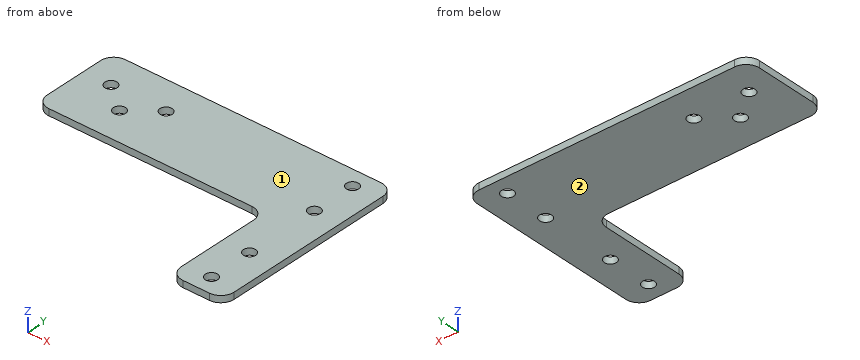
```python
from build123d import *

# Parameters (mm, degrees)
ODGI_CIE_BAZOWE1_DEPTH = 3
OTW_R_POD_RUB_M51_D    = 5.5
ZAOKR_GLENIE1_R        = 6


# Sheet-metal steps are written as plain solids
with BuildPart() as part:
    # Szkic1 → Odgięcie bazowe1 (new body)
    with BuildSketch(Plane.XY):
        Polygon((0, 0), (-104, 0), (-104, 40), (24, 40), (24, -50), (0, -50), align=None)
    extrude(amount=-ODGI_CIE_BAZOWE1_DEPTH)

    # Otwór pod śrubę M51 (through all)
    with Locations(Plane.XY):
        with Locations((12, -42), (12, -22), (12, 12), (12, 32), (-91.5, 25), (-66.5, 25), (-79, 15)):
            Hole(OTW_R_POD_RUB_M51_D / 2)

    # Zaokrąglenie1
    zaokr_glenie1_edges = [part.edges().sort_by_distance(p)[0] for p in [
        (0, 0, -1.5),
        (-104, 0, -1.5),
        (-104, 40, -1.5),
        (24, 40, -1.5),
        (24, -50, -1.5),
        (0, -50, -1.5),
    ]]
    fillet(zaokr_glenie1_edges, radius=ZAOKR_GLENIE1_R)


solid = part.part
```
The listing builds one solid part. Answer for the finished solid, in the listing's coordinates (mm). Face numbers are marked on the shaded views. Give positions to 0.01 mm unless a question says otherwise; leave off trailing zeros. Write each loop counter-clockwise with the first axis right and the second up, starting at its lowest first coordinate (ties: lowest second). Pieces come first, ordered by that corner, then holes. Notation, with made-up numbers: (54, 23) -> (72, 23) arc R29 cw to (72, 44) -> close; hole circle Ø11 at (-39.75, -5). An arc over 180 degrees is marked (long way). Write item = value, one per line. Start each with the question number.
1) The part is cut by section A-A, the plane y = 32. Determine the outline of the cut face in (x, z).
2) Each of these flat-tipped pins is pushed along its axis until it touches: pin 1 (0.9 mm diameter, centred on y = -25, z = -2, fed in from -X); pin 2 (0.9 mm diameter, centred on x = -45.5, z = -2, fed in from -Y). Where does it stop, or does it pass through?
3) The part is cut by section B-B, the plane x = -66.5. Determine the outline of the cut face in (y, z), and give its area (4 significant figures).
4) The part is cut by section D-D, the plane x = 12. Determine the outline of the cut face in (y, z), and give its area (3 significant figures).
5) The part is cut by section C-C, the plane z = -2.2. Determine the outline of the cut face in (x, y), and give its area (3 significant figures).
6) Determine the mould class of the marked faces 1 and 2 for opening direction Z: +Z half, -Z half, draft (parallel to the pull), parting line (faces both ways), or undercut.
7) Straight lines are drawn through the part: line 1 along Y through (x, z) = (12, -2.2); line 2 along Y through (x, z) = (-66.5, -1.75); line 3 along Y through (x, z) = (-21, -2.7). For each, find the intervals that lie inside material, in ascending order.
Solutions:
q1.outline = (-104, -3) -> (9.25, -3) -> (9.25, 0) -> (-104, 0) -> close; (14.75, -3) -> (24, -3) -> (24, 0) -> (14.75, 0) -> close
q2.pin_1 = 0
q2.pin_2 = 0
q3.outline = (0, -3) -> (22.25, -3) -> (22.25, 0) -> (0, 0) -> close; (27.75, -3) -> (40, -3) -> (40, 0) -> (27.75, 0) -> close
q3.area = 103.5 mm²
q4.outline = (-50, -3) -> (-44.75, -3) -> (-44.75, 0) -> (-50, 0) -> close; (-39.25, -3) -> (-24.75, -3) -> (-24.75, 0) -> (-39.25, 0) -> close; (-19.25, -3) -> (9.25, -3) -> (9.25, 0) -> (-19.25, 0) -> close; (14.75, -3) -> (29.25, -3) -> (29.25, 0) -> (14.75, 0) -> close; (34.75, -3) -> (40, -3) -> (40, 0) -> (34.75, 0) -> close
q4.area = 204 mm²
q5.outline = (-104, 6) arc R6 ccw to (-98, 0) -> (-6, 0) arc R6 cw to (0, -6) -> (0, -44) arc R6 ccw to (6, -50) -> (18, -50) arc R6 ccw to (24, -44) -> (24, 34) arc R6 ccw to (18, 40) -> (-98, 40) arc R6 ccw to (-104, 34) -> close; hole circle Ø5.5 at (-91.5, 25); hole circle Ø5.5 at (-79, 15); hole circle Ø5.5 at (-66.5, 25); hole circle Ø5.5 at (12, -42); hole circle Ø5.5 at (12, -22); hole circle Ø5.5 at (12, 12); hole circle Ø5.5 at (12, 32)
q5.area = 6,120 mm²
q6.face_1 = +Z half
q6.face_2 = -Z half
q7.line_1 = -50 to -44.75, -39.25 to -24.75, -19.25 to 9.25, 14.75 to 29.25, 34.75 to 40
q7.line_2 = 0 to 22.25, 27.75 to 40
q7.line_3 = 0 to 40
